```python
from build123d import *

# Parameters (mm, degrees)
SKETCH1_W                       = 140
SKETCH1_H                       = 80
BOSS_EXTRUDE1_DEPTH             = 2
CHAMFER2_SIZE                   = 2
SKETCH4_W                       = 8
SKETCH4_H                       = 10
BOSS_EXTRUDE2_DEPTH             = 7
SKETCH5_R                       = 2.05
CUT_EXTRUDE1_DEPTH              = 139.965499445
SKETCH6_W                       = 107.8
SKETCH6_H                       = 64
CUT_EXTRUDE2_DEPTH              = 5
SKIZZE1_R                       = 2.15
SCHNITT_LINEAR_AUSTRAGEN2_DEPTH = 10
SKIZZE2_W                       = 14.3
SKIZZE2_H                       = 14.3
SKIZZE2_R                       = 3.2
AUFSATZ_LINEAR_AUSTRAGEN1_DEPTH = 2
SKIZZE2_4_R                     = 3.2
SCHNITT_LINEAR_AUSTRAGEN4_DEPTH = 10
SKIZZE5_R                       = 2.15
AUFSATZ_LINEAR_AUSTRAGEN2_DEPTH = 2
SKIZZE4_R                       = 3.65
SKIZZE4_R_2                     = 2.05
AUFSATZ_LINEAR_AUSTRAGEN3_DEPTH = 10


with BuildPart() as part:
    # Sketch1 → Boss-Extrude1 (new body)
    with BuildSketch(Plane(origin=(0, 0, 0), x_dir=(1, 0, 0), z_dir=(0, 1, 0))):
        Rectangle(SKETCH1_W, SKETCH1_H)
    extrude(amount=BOSS_EXTRUDE1_DEPTH)

    # Sketch3 → Loft1 section 0
    with BuildSketch(Plane(origin=(0, 7, 0), x_dir=(1, 0, 0), z_dir=(0, 1, 0))):
        with BuildLine():
            Line((-63, -33), (63, -33))
            Line((63, -33), (63, 33))
            Line((63, 33), (-63, 33))
            Line((-63, 33), (-63, -33))
        make_face()
    # Sketch2 → Loft1 section 1
    with BuildSketch(Plane(origin=(0, 2, 0), x_dir=(1, 0, 0), z_dir=(0, 1, 0))):
        with BuildLine():
            Line((70, -40), (70, 40))
            Line((70, 40), (-70, 40))
            Line((-70, 40), (-70, -40))
            Line((-70, -40), (70, -40))
        make_face()
    loft()

    # Chamfer2
    chamfer2_edges = [part.edges().sort_by_distance(p)[0] for p in [
        (70, 1, 40),
        (-70, 1, 40),
        (-70, 1, -40),
        (70, 1, -40),
    ]]
    chamfer(chamfer2_edges, length=CHAMFER2_SIZE)

    # Sketch4 → Boss-Extrude2 (add)
    with BuildSketch(Plane.XZ):
        with Locations((-58.9, 20)):
            Rectangle(SKETCH4_W, SKETCH4_H)
        with Locations((-58.9, -20)):
            Rectangle(SKETCH4_W, SKETCH4_H)
        with Locations((58.9, -20)):
            Rectangle(SKETCH4_W, SKETCH4_H)
        with Locations((58.9, 20)):
            Rectangle(SKETCH4_W, SKETCH4_H)
    extrude(amount=BOSS_EXTRUDE2_DEPTH)

    # Sketch5 → Cut-Extrude1 (cut, through all)
    with BuildSketch(Plane.ZY.offset(62.9)):
        with Locations((-20, -3.5)):
            Circle(SKETCH5_R)
        with Locations((20, -3.5)):
            Circle(SKETCH5_R)
    extrude(amount=-CUT_EXTRUDE1_DEPTH, mode=Mode.SUBTRACT)

    # Sketch6 → Cut-Extrude2 (cut)
    with BuildSketch(Plane.XZ):
        Rectangle(SKETCH6_W, SKETCH6_H)
    extrude(amount=-CUT_EXTRUDE2_DEPTH, mode=Mode.SUBTRACT)

    # Skizze1 → Schnitt-Linear austragen2 (cut)
    with BuildSketch(Plane(origin=(0, 7, 0), x_dir=(1, 0, 0), z_dir=(0, 1, 0))):
        with Locations(Location((-50, -25, 0), (0, 0, 270))):
            Circle(SKIZZE1_R)
        with Locations(Location((-40, -25, 0), (0, 0, 270))):
            Circle(SKIZZE1_R)
        with Locations(Location((-30, -25, 0), (0, 0, 270))):
            Circle(SKIZZE1_R)
        with Locations(Location((-20, -25, 0), (0, 0, 270))):
            Circle(SKIZZE1_R)
        with Locations(Location((-10, -25, 0), (0, 0, 270))):
            Circle(SKIZZE1_R)
        with Locations(Location((0, -25, 0), (0, 0, 270))):
            Circle(SKIZZE1_R)
        with Locations(Location((10, -25, 0), (0, 0, 270))):
            Circle(SKIZZE1_R)
        with Locations(Location((20, -25, 0), (0, 0, 270))):
            Circle(SKIZZE1_R)
        with Locations(Location((30, -25, 0), (0, 0, 270))):
            Circle(SKIZZE1_R)
        with Locations(Location((40, -25, 0), (0, 0, 270))):
            Circle(SKIZZE1_R)
        with Locations(Location((50, -25, 0), (0, 0, 270))):
            Circle(SKIZZE1_R)
        with Locations(Location((-40, -15, 0), (0, 0, 270))):
            Circle(SKIZZE1_R)
        with Locations(Location((-30, -15, 0), (0, 0, 270))):
            Circle(SKIZZE1_R)
        with Locations(Location((-20, -15, 0), (0, 0, 270))):
            Circle(SKIZZE1_R)
        with Locations(Location((-10, -15, 0), (0, 0, 270))):
            Circle(SKIZZE1_R)
        with Locations(Location((0, -15, 0), (0, 0, 270))):
            Circle(SKIZZE1_R)
        with Locations(Location((10, -15, 0), (0, 0, 270))):
            Circle(SKIZZE1_R)
        with Locations(Location((20, -15, 0), (0, 0, 270))):
            Circle(SKIZZE1_R)
        with Locations(Location((30, -15, 0), (0, 0, 270))):
            Circle(SKIZZE1_R)
        with Locations(Location((40, -15, 0), (0, 0, 270))):
            Circle(SKIZZE1_R)
        with Locations(Location((50, -15, 0), (0, 0, 270))):
            Circle(SKIZZE1_R)
        with Locations(Location((-40, -5, 0), (0, 0, 270))):
            Circle(SKIZZE1_R)
        with Locations(Location((-30, -5, 0), (0, 0, 270))):
            Circle(SKIZZE1_R)
        with Locations(Location((-20, -5, 0), (0, 0, 270))):
            Circle(SKIZZE1_R)
        with Locations(Location((-10, -5, 0), (0, 0, 270))):
            Circle(SKIZZE1_R)
        with Locations(Location((0, -5, 0), (0, 0, 270))):
            Circle(SKIZZE1_R)
        with Locations(Location((10, -5, 0), (0, 0, 270))):
            Circle(SKIZZE1_R)
        with Locations(Location((20, -5, 0), (0, 0, 270))):
            Circle(SKIZZE1_R)
        with Locations(Location((30, -5, 0), (0, 0, 270))):
            Circle(SKIZZE1_R)
        with Locations(Location((40, -5, 0), (0, 0, 270))):
            Circle(SKIZZE1_R)
        with Locations(Location((50, -5, 0), (0, 0, 270))):
            Circle(SKIZZE1_R)
        with Locations(Location((-40, 5, 0), (0, 0, 270))):
            Circle(SKIZZE1_R)
        with Locations(Location((-30, 5, 0), (0, 0, 270))):
            Circle(SKIZZE1_R)
        with Locations(Location((-20, 5, 0), (0, 0, 270))):
            Circle(SKIZZE1_R)
        with Locations(Location((-10, 5, 0), (0, 0, 270))):
            Circle(SKIZZE1_R)
        with Locations(Location((0, 5, 0), (0, 0, 270))):
            Circle(SKIZZE1_R)
        with Locations(Location((10, 5, 0), (0, 0, 270))):
            Circle(SKIZZE1_R)
        with Locations(Location((20, 5, 0), (0, 0, 270))):
            Circle(SKIZZE1_R)
        with Locations(Location((30, 5, 0), (0, 0, 270))):
            Circle(SKIZZE1_R)
        with Locations(Location((40, 5, 0), (0, 0, 270))):
            Circle(SKIZZE1_R)
        with Locations(Location((50, 5, 0), (0, 0, 270))):
            Circle(SKIZZE1_R)
        with Locations(Location((-40, 15, 0), (0, 0, 270))):
            Circle(SKIZZE1_R)
        with Locations(Location((-30, 15, 0), (0, 0, 270))):
            Circle(SKIZZE1_R)
        with Locations(Location((-20, 15, 0), (0, 0, 270))):
            Circle(SKIZZE1_R)
        with Locations(Location((-10, 15, 0), (0, 0, 270))):
            Circle(SKIZZE1_R)
        with Locations(Location((0, 15, 0), (0, 0, 270))):
            Circle(SKIZZE1_R)
        with Locations(Location((10, 15, 0), (0, 0, 270))):
            Circle(SKIZZE1_R)
        with Locations(Location((20, 15, 0), (0, 0, 270))):
            Circle(SKIZZE1_R)
        with Locations(Location((30, 15, 0), (0, 0, 270))):
            Circle(SKIZZE1_R)
        with Locations(Location((40, 15, 0), (0, 0, 270))):
            Circle(SKIZZE1_R)
        with Locations(Location((50, 15, 0), (0, 0, 270))):
            Circle(SKIZZE1_R)
        with Locations(Location((-40, 25, 0), (0, 0, 270))):
            Circle(SKIZZE1_R)
        with Locations(Location((-30, 25, 0), (0, 0, 270))):
            Circle(SKIZZE1_R)
        with Locations(Location((-20, 25, 0), (0, 0, 270))):
            Circle(SKIZZE1_R)
        with Locations(Location((-10, 25, 0), (0, 0, 270))):
            Circle(SKIZZE1_R)
        with Locations(Location((0, 25, 0), (0, 0, 270))):
            Circle(SKIZZE1_R)
        with Locations(Location((10, 25, 0), (0, 0, 270))):
            Circle(SKIZZE1_R)
        with Locations(Location((20, 25, 0), (0, 0, 270))):
            Circle(SKIZZE1_R)
        with Locations(Location((30, 25, 0), (0, 0, 270))):
            Circle(SKIZZE1_R)
        with Locations(Location((40, 25, 0), (0, 0, 270))):
            Circle(SKIZZE1_R)
        with Locations(Location((50, 25, 0), (0, 0, 270))):
            Circle(SKIZZE1_R)
        with Locations(Location((-50, -15, 0), (0, 0, 270))):
            Circle(SKIZZE1_R)
        with Locations(Location((-50, -5, 0), (0, 0, 270))):
            Circle(SKIZZE1_R)
        with Locations(Location((-50, 5, 0), (0, 0, 270))):
            Circle(SKIZZE1_R)
        with Locations(Location((-50, 15, 0), (0, 0, 270))):
            Circle(SKIZZE1_R)
        with Locations(Location((-50, 25, 0), (0, 0, 270))):
            Circle(SKIZZE1_R)
    extrude(amount=-SCHNITT_LINEAR_AUSTRAGEN2_DEPTH, mode=Mode.SUBTRACT)

    # Skizze2 → Aufsatz-Linear austragen1 (add)
    with BuildSketch(Plane(origin=(0, 7, 0), x_dir=(1, 0, 0), z_dir=(0, 1, 0))):
        with Locations((45, -20)):
            Rectangle(SKIZZE2_W, SKIZZE2_H)
        with Locations((45, -20)):
            Circle(SKIZZE2_R, mode=Mode.SUBTRACT)
    extrude(amount=-AUFSATZ_LINEAR_AUSTRAGEN1_DEPTH)

    # Skizze2<4> → Schnitt-Linear austragen4 (cut)
    with BuildSketch(Plane(origin=(0, 7, 0), x_dir=(1, 0, 0), z_dir=(0, 1, 0))):
        with Locations(Location((45, -20, 0), (0, 0, 270))):
            Circle(SKIZZE2_4_R)
    extrude(amount=-SCHNITT_LINEAR_AUSTRAGEN4_DEPTH, mode=Mode.SUBTRACT)

    # Skizze5 → Aufsatz-Linear austragen2 (add)
    with BuildSketch(Plane(origin=(0, 7, 0), x_dir=(1, 0, 0), z_dir=(0, 1, 0))):
        with Locations((20, -15)):
            Circle(SKIZZE5_R)
        with Locations((20, 15)):
            Circle(SKIZZE5_R)
        with Locations((-20, 15)):
            Circle(SKIZZE5_R)
        with Locations((-20, -15)):
            Circle(SKIZZE5_R)
    extrude(amount=-AUFSATZ_LINEAR_AUSTRAGEN2_DEPTH)

    # Skizze4 → Aufsatz-Linear austragen3 (add)
    # profile 1 of 4: a face of its own
    with BuildSketch(Plane(origin=(0, 7, 0), x_dir=(1, 0, 0), z_dir=(0, 1, 0))):
        with Locations(Location((-23.105, 17.725, 0), (0, 0, 270))):
            Circle(SKIZZE4_R)
        with Locations(Location((-23.105, 17.725, 0), (0, 0, 270))):
            Circle(SKIZZE4_R_2, mode=Mode.SUBTRACT)
    # profile 2 of 4: a face of its own
    with BuildSketch(Plane(origin=(0, 7, 0), x_dir=(1, 0, 0), z_dir=(0, 1, 0))):
        with Locations(Location((23.105, 17.725, 0), (0, 0, 270))):
            Circle(SKIZZE4_R)
        with Locations(Location((23.105, 17.725, 0), (0, 0, 270))):
            Circle(SKIZZE4_R_2, mode=Mode.SUBTRACT)
    # profile 3 of 4: a face of its own
    with BuildSketch(Plane(origin=(0, 7, 0), x_dir=(1, 0, 0), z_dir=(0, 1, 0))):
        with Locations(Location((23.105, -17.725, 0), (0, 0, 270))):
            Circle(SKIZZE4_R)
        with Locations(Location((23.105, -17.725, 0), (0, 0, 270))):
            Circle(SKIZZE4_R_2, mode=Mode.SUBTRACT)
    # profile 4 of 4: a face of its own
    with BuildSketch(Plane(origin=(0, 7, 0), x_dir=(1, 0, 0), z_dir=(0, 1, 0))):
        with Locations(Location((-23.105, -17.725, 0), (0, 0, 270))):
            Circle(SKIZZE4_R)
        with Locations(Location((-23.105, -17.725, 0), (0, 0, 270))):
            Circle(SKIZZE4_R_2, mode=Mode.SUBTRACT)
    extrude(amount=-AUFSATZ_LINEAR_AUSTRAGEN3_DEPTH)


solid = part.part
```
Here's how the part is built. I have some questions about the finished solid (model axes, mm). A direction names the side the tool comes from. Round coordinates to 2 decimals unless told otherwise and drop trailing zeros.
Q1. Will these pins go through, and if not, where does the flat tip stop? P1, Ø5.5, axis at x = 20, z = -5, coming from the -Y side; P2, Ø3.5, axis at x = -30, z = 5, coming from the +Y side; P3, Ø2, axis at y = -5, z = -20.5, coming from the +X side; P4, Ø1.5, axis at y = 3, z = -30, coming from the -X side.
Q2. Which directions (+Z, -Z, +X, -X, +Y, -Y) give clear straight access to the entire face, cutting with the end or side of a thin tool? Please do faces 1 (the flat face through (-1, 5, 0)), 2 (the flat face through (-59, -3, 25)), 3 (the flat face through (-54.9, -3.5, 17.7)), 4 (the cylindrical face through (18.09, 6.01, -24.01)).
Q3. If we section it at A-A on x = 40: Give the number of separate pieces and of enclosed holes in the cut face, plus the area to 3 significant figures.
Q4. If we mould it in two halves opening along X, with no side actions, what happens to faces 5 (the cylindrical face through (21.71, 1.06, 21.1)), 6 (the flat face through (-62.9, -3.5, 17.7)), 7 (the flat face through (62.9, -3.5, -22.3))? For each: +X half, -X half, draft (parallel to the pull), parting line (faces both ways), or undercut.
Q5. Please list where these lines run through material, in increasing order: probe 1 along X at (y, z) = (0.25, 25); probe 2 along Z at (x, y) = (27.5, 0.25); probe 3 along Z at (x, y) = (55, -0.5).
Answer below:
1. P1: stops at y = 5
1. P2: passes through
1. P3: stops at x = 62.9
1. P4: stops at x = -69.65
2. face 1: -Y
2. face 2: +Z, +X, -X, -Y
2. face 3: +Z, -Z, -Y
2. face 4: +Y, -Y
3. separate pieces: 5
3. enclosed holes: 0
3. area: 171 mm2
4. face 5: undercut
4. face 6: -X half
4. face 7: +X half
5. probe 1: x = -70 to -53.9, 53.9 to 70
5. probe 2: z = -40 to -32, 32 to 40
5. probe 3: z = -25 to -15, 15 to 25
